```python
from build123d import *

# Parameters (mm, degrees)
SKETCH_1_W             = 50
SKETCH_1_H             = 5
BLOCKEXTRUDE_DEPTH     = 70
FILLET_2_R             = 3
SKETCH_2_R             = 8
ROTARY_SEAL_SEAT_DEPTH = 87.168439698


with BuildPart() as part:
    # 草图1 → BlockExtrude (new body)
    with BuildSketch(Plane.XY):
        with Locations((25, 2.5)):
            Rectangle(SKETCH_1_W, SKETCH_1_H)
    extrude(amount=BLOCKEXTRUDE_DEPTH)

    # Fillet 2
    fillet_2_edges = [part.edges().sort_by_distance(p)[0] for p in [
        (50, 2.5, 70),
        (0, 2.5, 70),
        (50, 2.5, 0),
        (0, 2.5, 0),
    ]]
    fillet(fillet_2_edges, radius=FILLET_2_R)

    # 草图2 → Rotary_seal_seat (cut, through all)
    with BuildSketch(Plane(origin=(0, 5, 0), x_dir=(1, 0, 0), z_dir=(0, 1, 0))):
        with Locations(Location((25, -45, 0), (0, 0, 270))):
            Circle(SKETCH_2_R)
    extrude(amount=-ROTARY_SEAL_SEAT_DEPTH, mode=Mode.SUBTRACT)


solid = part.part
```
Read the model definition and answer for the solid it produces. Units are mm, in the model's axes. Coordinates: 2 decimals unless noted, no trailing zeros. Write each loop counter-clockwise with the first axis right and the second up, starting at its lowest first coordinate (ties: lowest second). Pieces come first, ordered by that corner, then holes. Notation, with made-up numbers: (-19.5, -39.5) -> (31.5, -39.5) arc R36 ccw to (31.5, -0.5) -> close; hole circle Ø2 at (-34.75, 45.25). An arc over 180 degrees is marked (long way). Return JSON: item names as keys, results as strings.
1. This flat-tipped pin is pushed along its axis until it touches: P1, Ø5, axis at x = 15, z = 13, coming from the -Y side. Where does it stop, or does it pass through?
Found:
{"P1": "y = 0"}
2. Determine the mould class of faces 1 (the face through (49.14, 2.54, 69.1)), 2 (the face through (0.86, 2.54, 69.1)), 3 (the face through (25, 3, 70)), 4 (the face through (30.4, 2.5, 39.1)) for opening direction X: pulls with the +X half, pulls with the -X half, needs draft (parallel to the pull), parting line crosses it, or undercut.
Found:
{"face 1": "pulls with the +X half", "face 2": "pulls with the -X half", "face 3": "needs draft", "face 4": "undercut"}
3. A cutting plane is placed at A-A (z = 45). Determine the outline of the cut face in (x, y).
Found:
{"outline": "(0, 0) -> (17, 0) -> (17, 5) -> (0, 5) -> close; (33, 0) -> (50, 0) -> (50, 5) -> (33, 5) -> close"}
4. A cutting plane is placed at B-B (x = 25). Determine the outline of the cut face in (y, z).
Found:
{"outline": "(0, 0) -> (5, 0) -> (5, 37) -> (0, 37) -> close; (0, 53) -> (5, 53) -> (5, 70) -> (0, 70) -> close"}
5. Find the intervals of material crossed by line 1 along X through (y, z) = (3.45, 45); line 2 along X through (y, z) = (2.05, 51), in increasing order. Write a range as from..to.
Found:
{"line 1": "0..17, 33..50", "line 2": "0..19.71, 30.29..50"}
6. A cutting plane is placed at C-C (y = 1.4). Determine the outline of the cut face in (x, z), and give its area (3 significant figures).
Found:
{"outline": "(0, 3) arc R3 ccw to (3, 0) -> (47, 0) arc R3 ccw to (50, 3) -> (50, 67) arc R3 ccw to (47, 70) -> (3, 70) arc R3 ccw to (0, 67) -> close; hole circle Ø16 at (25, 45)", "area": "3,290 mm2"}
